The model under review builds one solid part; all positions refer to its coordinate system, in mm. A direction names the side the tool comes from. Round coordinates to 2 decimals unless told otherwise and drop trailing zeros. Order: outer loops, then holes, each group sorted by start corner. A loop starts at its lowest first (then second) coordinate and runs counter-clockwise, first axis right, second up. Notation, with made-up numbers: M 6.5,-2.5 L 52.5,-2.5 A27 ccw 52.5,20.5 Z; hole C -39,19 d9. An arc over 180 degrees is marked long. Answer as a JSON object with one key per item and string values. Group by question number.
1. Add section A-A on z = 8.75. State the section outline as (x, y) points.
2. To check wall thickness, follow probe 1 along Z at (x, y) = (-5.5, -4.5); probe 2 along Z at (x, y) = (-26, -0.5); probe 3 along X at (y, z) = (-16.5, 2). State the ranges of each line that lie inside material, in increasing order. Write a range as [from, to].
3. Clearance check with flat-ended pins moving along their axes: P1, Ø6, axis at y = 23, z = 3, coming from the -X side; P2, Ø1, axis at y = -0.5, z = 3.5, coming from the -X side; P3, Ø6, axis at x = -11, z = 6, coming from the -Y side. State where each tip first meets the part, or that it passes through.
4. Machinability: for faces 4 (the face through (16, -18, 0)), 5 (the face through (-18.87, 17.3, 9.39)), which of the approach directions +Z, -Z, +X, -X, +Y, -Y give a long, thin tool a straight path to every point of the face, cutting with its end or side? Answer none if there is none.
5. Mouldability with a two-part tool opening along Y and no side actions: class faces 1 (the face through (0, 0, 4)), 2 (the face through (23.5, 10.7, 6.7)), 3 (the face through (-7.69, -34.61, 5.84)) as released by +Y, released by -Y, zero draft, split by the parting line, or undercut.
```python
from build123d import *

# Parameters (mm, degrees)
F0_R     = 35.4529924148
F0_R_2   = 26.5998947574
F1_DEPTH = 12
F2_R     = 20.3647706408
F3_DEPTH = 4
F5_R     = 5
F6_R     = 5
F7_R     = 35.4529924148
F7_R_2   = 25.6021329211
F8_DEPTH = 5.3


# Not quite as in the source:
# - a fillet or chamfer that OpenCascade refuses, or shapes differently, is made with other operations: its cross-section is extruded or revolved along the edge and cut away or added


with BuildPart() as f1:
    # F0 (on Top) → F1 (new body)
    with BuildSketch(Plane.XY):
        Circle(F0_R)
        Circle(F0_R_2, mode=Mode.SUBTRACT)
        Circle(F0_R_2)
    extrude(amount=F1_DEPTH)

    # F2 (on face) → F3 (cut)
    with BuildSketch(Plane(origin=(0, 0, 0), x_dir=(1, 0, 0), z_dir=(0, 0, -1))):
        Circle(F2_R)
    extrude(amount=-F3_DEPTH, mode=Mode.SUBTRACT)

    # F4: fillet of radius 5 on 1 edges, made by hand

    # F4_s1 → F4_t2 (revolve)
    with BuildSketch(Plane.XZ):
        with BuildLine():
            ThreePointArc((20.3647706408, 0), (18.6280688154, 2.8729833462), (15.4657911552, 4))
            Line((15.4657911552, 4), (20.3647706408, 4))
            Line((20.3647706408, 4), (20.3647706408, 0))
        make_face()
    revolve(axis=Axis((0, 0, 4), (0, 0, -1)))

    # F5
    f5_edges = [f1.edges().sort_by_distance(p)[0] for p in [
        (-20.364771, 0, 0),
    ]]
    fillet(f5_edges, radius=F5_R)

    # F6
    f6_edges = [f1.edges().sort_by_distance(p)[0] for p in [
        (-35.452992, 0, 0),
    ]]
    fillet(f6_edges, radius=F6_R)

    # F7 (on face) → F8 (cut)
    with BuildSketch(Plane.XY.offset(12)):
        Circle(F7_R)
        Circle(F7_R_2, mode=Mode.SUBTRACT)
    extrude(amount=-F8_DEPTH, mode=Mode.SUBTRACT)


solid = f1.part
```
Recorded:
{
 "1": {"outline": "C 0,0 d51.2"},
 "2": {"probe 1": "z = [4, 12]", "probe 2": "z = [0, 6.7]", "probe 3": "x = [-30.24, -10.33], [10.33, 30.24]"},
 "3": {"P1": "stops at x = -29.03", "P2": "stops at x = -35.35", "P3": "stops at y = -34.54"},
 "4": {"face 4": "-Z, +X, -X, +Y, -Y", "face 5": "+Z"},
 "5": {"face 1": "undercut", "face 2": "zero draft", "face 3": "split by the parting line"}
}
